Verification items for the finished model (mm, model axes). A direction names the side the tool comes from. Coordinates: 2 decimals unless noted, no trailing zeros. Loops run counter-clockwise (first coordinate to the right, second up) from the corner with the lowest first, then second, coordinate; pieces in that order, holes last. Notation, with made-up numbers: (81, -15.5) -> (108, -15.5) arc R17 ccw to (108, 7.5) -> close; hole circle Ø10 at (67, 89.25). An arc over 180 degrees is marked (long way). Answer as a JSON object with one key per item and string values. Group by question number.
Q1. Release check for a two-part mould opening along X. For faces 1 (the cylindrical face through (-2.333, 7.207, 1.536)), 2 (the flat face through (0, 0, 2)), 3 (the flat face through (0.813, 8.48, 2.893)) record: released by +X, released by -X, zero draft, split by the parting line, or undercut.
Q2. Cross-section at D-D on y = 11.75. Record the boundary of the cut face in (x, z), and give its area (3 significant figures).
Q3. Cross-section at C-C on z = 1.75. Record the boundary of the cut face in (x, y).
Q4. Gauge pin test, flat ends, axial feed: pin 1 Ø1.5 at (x, y) = (-5, 5.5) entering from +Z; pin 2 Ø4 at (y, z) = (4.5, -2) entering from +X; pin 3 Ø3 at (x, z) = (-4, 1.5) entering from +Y. Record the tip position at first contact, or that the pin passes through.
Q5. Cross-section at B-B on y = 2.5. Record the boundary of the cut face in (x, z).
Q6. Set-up check for faces 4 (the cylindrical face through (0, 3, -4)), 5 (the cylindrical face through (-1.464, 4.135, 0.325)): record each of +Z, -Z, +X, -X, +Y, -Y from which the full face is reachable in a straight line by a thin tool's end or side.
Q7. Cross-section at A-A on z = 0. Record the boundary of the cut face in (x, y).
Q8. Scan lines: L1, parallel to Z at x = 0, y = 3; L2, parallel to Z at x = 0, y = 4.5. Record each from-to range of solid material in increasing order.
```python
from build123d import *

# Parameters (mm, degrees)
SKETCH1_R               = 4
BOSS_EXTRUDE1_DEPTH     = 10
CUT_EXTRUDE1_DEPTH      = 21.928449536
CUT_EXTRUDE1_DEPTH_BACK = 21.928449536
SKETCH9_R               = 1.5
CUT_EXTRUDE5_DEPTH      = 19.276446179
SKETCH7_R               = 1.5
CUT_EXTRUDE3_DEPTH      = 20.008489752


with BuildPart() as part:
    # Sketch1 → Boss-Extrude1 (new body)
    with BuildSketch(Plane(origin=(0, 0, 0), x_dir=(1, 0, 0), z_dir=(0, 1, 0))):
        with Locations(Location((0, 0, 0), (0, 0, 270))):
            Circle(SKETCH1_R)
    extrude(amount=BOSS_EXTRUDE1_DEPTH)

    # Sketch2 → Revolve2 (revolve)
    with BuildSketch(Plane(origin=(0, 0, 0), x_dir=(0, 0, -1), z_dir=(1, 0, 0))):
        with BuildLine():
            Line((-3, 3), (-3, 17))
            ThreePointArc((-3, 17), (4, 10), (-3, 3))
        make_face()
    revolve(axis=Axis((0, 3, 3), (0, 1, 0)))

    # Sketch5 → Cut-Extrude1 (cut, two sides: drawn at the far end of the back side and taken through both)
    with BuildSketch(Plane.XY.offset(-CUT_EXTRUDE1_DEPTH_BACK)):
        Polygon((-7, 17), (7, 17), (7, 3), (6.646446609, 2.646446609), (-7.353553391, 16.646446609), align=None)
    extrude(amount=CUT_EXTRUDE1_DEPTH + CUT_EXTRUDE1_DEPTH_BACK, mode=Mode.SUBTRACT)

    # Sketch9 → Cut-Extrude5 (cut, through all)
    with BuildSketch(Plane(origin=(4.646446609, 4.646446609, 0), x_dir=(0, 0, -1), z_dir=(0.7071067811865462, 0.7071067811865489, 0))):
        with Locations(Location((-3, 7.071067812, 0), (0, 0, 90))):
            Circle(SKETCH9_R)
    extrude(amount=-CUT_EXTRUDE5_DEPTH, mode=Mode.SUBTRACT)

    # Sketch7 → Cut-Extrude3 (cut, through all)
    with BuildSketch(Plane.XZ):
        with Locations(Location((0, 0, 0), (0, 0, 270))):
            Circle(SKETCH7_R)
    extrude(amount=-CUT_EXTRUDE3_DEPTH, mode=Mode.SUBTRACT)


solid = part.part
```
Computed values:
{
 "1": {"face 1": "undercut", "face 2": "zero draft", "face 3": "released by +X"},
 "2": {"outline": "(-2.46, -3.32) -> (-2.46, 9.32) arc R6.78 ccw to start", "area": "39.6 mm²"},
 "3": {"outline": "(-5.42, 5.75) -> (-0.94, 10.23) -> (-5.21, 14.5) arc R6.89 ccw to start; (-4.25, 4.58) arc R6.89 ccw to (-3.6, 4.13) -> (-3.6, 0) -> (3.6, 0) -> (3.6, 4.13) arc R6.89 ccw to (4.5, 4.79) -> (0.23, 9.06) -> close"},
 "4": {"pin 1": "stops at z = 6.64", "pin 2": "stops at x = 4.06", "pin 3": "stops at y = 14.56"},
 "5": {"outline": "circle Ø8 at (0, 0); hole circle Ø3 at (0, 0)"},
 "6": {"face 4": "-Y", "face 5": "+Y, -Y"},
 "7": {"outline": "(-4.81, 14.1) arc R6.32 ccw to (-4, 5.1) -> (-4, 0) -> (-1.5, 0) -> (-1.5, 10.79) -> close; (1.5, 0) -> (4, 0) -> (4, 5.1) arc R6.32 ccw to (4.1, 5.19) -> (1.5, 7.79) -> close"},
 "8": {"L1": "z = -4 to -1.5, 1.5 to 4", "L2": "z = -4 to -1.5, 1.5 to 7.33"}
}
